CAD build for the part. Positions are in the model's coordinates, mm. A direction names the side the tool comes from. Coordinates: 2 decimals unless noted, no trailing zeros. Order: outer loops, then holes, each group sorted by start corner. A loop starts at its lowest first (then second) coordinate and runs counter-clockwise, first axis right, second up. Notation, with made-up numbers: M 75,28 L 119,28 A22 cw 119,52 Z; hole C 3,89.25 d7. An arc over 180 degrees is marked long. Write item = value, one per line.
from build123d import *

# Parameters (mm, degrees)
BOSS_EXTRUDE1_DEPTH = 16.002


with BuildPart() as part:
    # Sketch1 → Revolve1 (revolve)
    with BuildSketch(Plane.XY):
        Polygon((-44.45, -84.1375), (28.448, -84.1375), (28.448, -91.2495), (44.45, -91.2495), (44.45, 0), (28.448, 0), (28.448, -77.0255), (-44.45, -77.0255), align=None)
    revolve(axis=Axis((-44.45, 0, 0), (1, 0, 0)))

    # Sketch2 → Boss-Extrude1 (add)
    with BuildSketch(Plane.ZY.offset(-28.448)):
        Polygon((-91.2495, 52.682923388), (-91.2495, -52.682923388), (0, -105.365846777), (91.2495, -52.682923388), (91.2495, 52.682923388), (0, 105.365846777), align=None)
    extrude(amount=-BOSS_EXTRUDE1_DEPTH)


solid = part.part
(1) Slice it at C-C, the plane z = -21.5. Write the cut outline in (x, y).
Evaluation:
outline = M -44.45,-81.34 L 28.45,-81.34 L 28.45,-92.95 L 44.45,-92.95 L 44.45,92.95 L 28.45,92.95 L 28.45,81.34 L -44.45,81.34 L -44.45,73.96 L 28.45,73.96 L 28.45,-73.96 L -44.45,-73.96 Z
(2) Slice it at B-B, the plane x = 36. Write the cut outline in (y, z).
Evaluation:
outline = M -105.37,0 L -52.68,-91.25 L 52.68,-91.25 L 105.37,0 L 52.68,91.25 L -52.68,91.25 Z
(3) Tool access for faces 4 (the face through (36.34, 79.39, -44.99)), 5 (the face through (28.448, -1, -1)): list every direction of +Z, -Z, +X, -X, +Y, -Y with a clear straight run to the whole face (end or side of a thin tool).
Evaluation:
face_4 = -Z, +X, -X, +Y
face_5 = -X
(4) Pin check, flat tips, straight feed: pin 1 Ø6 at (x, z) = (-22, -31.5) entering from -Y; pin 2 Ø3 at (x, z) = (10.5, 8.5) entering from -Y; pin 3 Ø2 at (x, z) = (-1.5, -51) entering from +Y. Stop position of each tip, or through.
Evaluation:
pin_1 = -79.16
pin_2 = -83.85
pin_3 = 67.67
(5) Wall check: line 1 (Z direction, x = -8, y = 0); line 2 (Z direction, x = 20, y = 7.5); line 3 (X direction, y = -52.5, z = -50). Give the ranges that are in metal, low to high. Write a range as from..to.
Evaluation:
line_1 = -84.14..-77.03, 77.03..84.14
line_2 = -83.8..-76.66, 76.66..83.8
line_3 = 28.45..44.45
(6) Slice it at A-A, the plane y = 0. Write the cut outline in (x, z), then the cut area to 3 significant figures.
Evaluation:
outline = M -44.45,-84.14 L 28.45,-84.14 L 28.45,-91.25 L 44.45,-91.25 L 44.45,91.25 L 28.45,91.25 L 28.45,84.14 L -44.45,84.14 L -44.45,77.03 L 28.45,77.03 L 28.45,-77.03 L -44.45,-77.03 Z
area = 3,960 mm²
(7) Pull direction Y, two halves, no side cores. Call faces 1 (the face through (-8.511, 16.698, 75.194)), 2 (the face through (-7.491, 18.239, 82.137)), 3 (the face through (-44.45, 37, 68)): +Y half, -Y half, draft (parallel to the pull), parting line (faces both ways), or undercut.
Evaluation:
face_1 = undercut
face_2 = parting line
face_3 = draft
(8) Slice it at D-D, the plane x = -28. Write the cut outline in (y, z) (1 decimal).
Evaluation:
outline = C 0,0 d168.3; hole C 0,0 d154.1
